Verification items for the finished model (mm, model axes). Face numbers are marked on the shaded views. A direction names the side the tool comes from. Coordinates: 2 decimals unless noted, no trailing zeros. Write each loop counter-clockwise with the first axis right and the second up, starting at its lowest first coordinate (ties: lowest second). Pieces come first, ordered by that corner, then holes. Notation, with made-up numbers: (25.5, 27) -> (80.5, 27) arc R24 cw to (80.5, 45) -> close; hole circle Ø9 at (8, 75.25). An arc over 180 degrees is marked (long way). Write item = value, one per line. Start each with the question number.
(1) Mould release check, pull along X, two halves, no side actions. Record for the marked faces 1, 2 and 3: released by +X, released by -X, zero draft, split by the parting line, or undercut.
(2) Gauge pin test, flat ends, axial feed: pin 1 Ø5 at (x, z) = (145, -8) entering from +Y; pin 2 Ø8 at (x, y) = (153.5, 53.5) entering from -Z; pin 3 Ø6 at (x, z) = (201.5, -1) entering from -Y; pin 4 Ø4 at (x, y) = (127.5, 61.5) entering from +Z. Record the tip position at first contact, or that the pin passes through.
(3) Material ranges on probe 1 along X at (y, z) = (67.25, 0); probe 2 along Z at (x, y) = (200, 43); probe 3 along X at (y, z) = (-4, 0), recorded low to high. Write a range as [from, to].
(4) Section check D-D (x = 59). Record the cut outline in (y, z) (3 decimals).
(5) Section check C-C (y = 57). Record the cut outline in (x, z), plus the area to 3 significant figures.
(6) Section check A-A (z = 0). Record the cut outline in (x, y), plus the area to 3 significant figures.
(7) Set-up check for the marked faces 4, 5, 6 and 7: record each of +Z, -Z, +X, -X, +Y, -Y from which the full face is reachable in a straight line by a thin tool's end or side.
(8) Section check B-B (x = 200). Record the cut outline in (y, z).
```python
from build123d import *

# Parameters (mm, degrees)
BOSS_EXTRUDE1_DEPTH     = 2
BOSS_EXTRUDE2_START     = -31.8
SKETCH3_W               = 60
SKETCH3_H               = 44
BOSS_EXTRUDE2_DEPTH     = 31.8
SKETCH4_R               = 4
BOSS_EXTRUDE3_DEPTH     = 7
CUT_EXTRUDE1_DEPTH      = 229.617169084
CUT_EXTRUDE1_DEPTH_BACK = 229.617169084
CUT_EXTRUDE2_DEPTH      = 228.560980838
CUT_EXTRUDE2_DEPTH_BACK = 228.560980838
SKETCH8_R               = 4.5
BOSS_EXTRUDE4_DEPTH     = 0.1


with BuildPart() as part:
    # Sketch1 → Boss-Extrude1 (new, symmetric)
    with BuildSketch(Plane.XY.offset(13.9)):
        Polygon((150, 27), (150, 71), (65.671641791, 44.328358209), (0, 0), (110, 0), align=None)
        Polygon((45.764296173, 14), (69.845614914, 30.25489015), (86.100505063, 14), align=None, mode=Mode.SUBTRACT)
        Polygon((84.347754219, 35.551740718), (136, 51.888477569), (136, 34.440899917), (105.826026877, 14.073468059), align=None, mode=Mode.SUBTRACT)
    extrude(amount=BOSS_EXTRUDE1_DEPTH, both=True)


with BuildPart() as body_2:
    # Mirror2: mirrored copy
    add(part.part.mirror(Plane.XY))


with BuildPart() as part_1:
    add(part.part)

    add(body_2.part)  # Boss-Extrude2 merges body 2
    # Sketch3 → Boss-Extrude2 (add)
    with BuildSketch(Plane.XY.offset(15.9).offset(BOSS_EXTRUDE2_START)):
        with Locations((180, 49)):
            Rectangle(SKETCH3_W, SKETCH3_H)
    extrude(amount=BOSS_EXTRUDE2_DEPTH)

    # Sketch4 → Boss-Extrude3 (add)
    with BuildSketch(Plane(origin=(0, 0, 0), x_dir=(1, 0, 0), z_dir=(0, 1, 0))):
        with BuildLine():
            Line((108.3763786, 39.867312377), (-1.6236214, 21.767312377))
            ThreePointArc((-1.6236214, 21.767312377), (-7.623523267, 18.37162213), (-10, 11.9))
            Line((-10, 11.9), (-10, -11.9))
            ThreePointArc((-10, -11.9), (-7.623523267, -18.37162213), (-1.6236214, -21.767312377))
            Line((-1.6236214, -21.767312377), (108.3763786, -39.867312377))
            ThreePointArc((108.3763786, -39.867312377), (116.47162213, -37.623523267), (120, -30))
            Line((120, -30), (120, 30))
            ThreePointArc((120, 30), (116.47162213, 37.623523267), (108.3763786, 39.867312377))
        make_face()
        with Locations(Location((110, 30, 0), (0, 0, 270))):
            Circle(SKETCH4_R, mode=Mode.SUBTRACT)
        with Locations(Location((110, -30, 0), (0, 0, 270))):
            Circle(SKETCH4_R, mode=Mode.SUBTRACT)
        with Locations(Location((0, 0, 0), (0, 0, 270))):
            Circle(SKETCH4_R, mode=Mode.SUBTRACT)
    extrude(amount=-BOSS_EXTRUDE3_DEPTH)

    # Sketch7 → Cut-Extrude1 (cut, two sides: drawn at the far end of the back side and taken through both)
    with BuildSketch(Plane.XY.offset(15.9).offset(-CUT_EXTRUDE1_DEPTH_BACK)):
        with BuildLine():
            Line((189.966629547, 50), (210, 50))
            Line((210, 50), (210, 48))
            Line((210, 48), (189.966629547, 48))
            ThreePointArc((189.966629547, 48), (160, 49), (189.966629547, 50))
        make_face()
    extrude(amount=CUT_EXTRUDE1_DEPTH + CUT_EXTRUDE1_DEPTH_BACK, mode=Mode.SUBTRACT)

    # Sketch8 → Cut-Extrude2 (cut, two sides: drawn at the far end of the back side and taken through both)
    with BuildSketch(Plane(origin=(0, 71, 0), x_dir=(1, 0, 0), z_dir=(0, 1, 0)).offset(-CUT_EXTRUDE2_DEPTH_BACK)):
        with Locations(Location((200, 0, 0), (0, 0, 270))):
            Circle(SKETCH8_R)
    extrude(amount=CUT_EXTRUDE2_DEPTH + CUT_EXTRUDE2_DEPTH_BACK, mode=Mode.SUBTRACT)

    # Sketch9 → Boss-Extrude4 (add)
    with BuildSketch(Plane.XY.offset(15.9)):
        with BuildLine():
            Line((150, 71), (150, 27))
            Line((150, 27), (210, 27))
            Line((210, 27), (210, 48))
            Line((210, 48), (189.966629547, 48))
            ThreePointArc((189.966629547, 48), (160, 49), (189.966629547, 50))
            Line((189.966629547, 50), (210, 50))
            Line((210, 50), (210, 71))
            Line((210, 71), (150, 71))
        make_face()
    extrude(amount=BOSS_EXTRUDE4_DEPTH)


solid = part_1.part
```
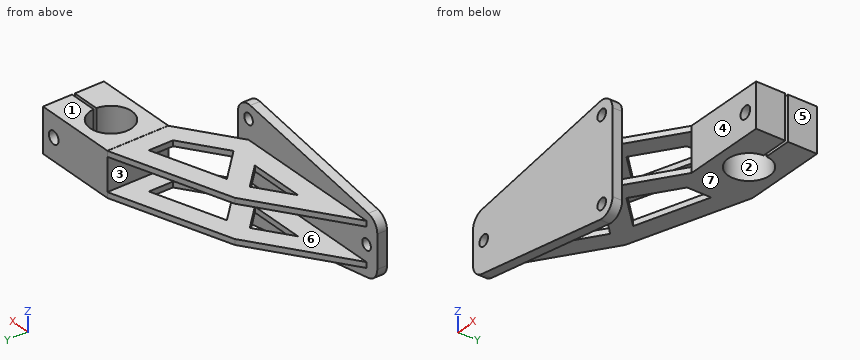
Response:
q1.face_1 = zero draft
q1.face_2 = undercut
q1.face_3 = released by -X
q2.pin_1 = through
q2.pin_2 = -15.9
q2.pin_3 = 27
q2.pin_4 = 15.9
q3.probe_1 = [150, 195.5], [204.5, 210]
q3.probe_2 = [-15.9, -4.5], [4.5, 16]
q3.probe_3 = [-10, -4], [4, 120]
q4.outline = (-7, -31.743) -> (0, -31.743) -> (0, -15.9) -> (14, -15.9) -> (14, -11.9) -> (0, -11.9) -> (0, 11.9) -> (14, 11.9) -> (14, 15.9) -> (0, 15.9) -> (0, 31.743) -> (-7, 31.743) -> close; (22.934, -15.9) -> (39.825, -15.9) -> (39.825, -11.9) -> (22.934, -11.9) -> close; (22.934, 11.9) -> (39.825, 11.9) -> (39.825, 15.9) -> (22.934, 15.9) -> close
q5.outline = (105.74, -15.9) -> (162.31, -15.9) -> (162.31, 16) -> (150, 16) -> (150, 15.9) -> (105.74, 15.9) -> (105.74, 11.9) -> (150, 11.9) -> (150, -11.9) -> (105.74, -11.9) -> close; (187.69, -15.9) -> (210, -15.9) -> (210, 16) -> (187.69, 16) -> close; hole circle Ø9 at (200, 0)
q5.area = 1,390 mm2
q6.outline = (-10, -7) -> (-4, -7) -> (-4, 0) -> (-10, 0) -> close; (4, -7) -> (120, -7) -> (120, 0) -> (4, 0) -> close; (150, 27) -> (195.5, 27) -> (195.5, 48) -> (189.97, 48) arc R15 cw (long way) to (189.97, 50) -> (195.5, 50) -> (195.5, 71) -> (150, 71) -> close; (204.5, 27) -> (210, 27) -> (210, 48) -> (204.5, 48) -> close; (204.5, 50) -> (210, 50) -> (210, 71) -> (204.5, 71) -> close
q6.area = 2,370 mm2
q7.face_4 = +Z, -Z, +X, -Y
q7.face_5 = +Z, -Z, +X, +Y, -Y
q7.face_6 = -X, +Y
q7.face_7 = -Z, +X, -X, +Y
q8.outline = (27, -15.9) -> (48, -15.9) -> (48, -4.5) -> (27, -4.5) -> close; (27, 4.5) -> (48, 4.5) -> (48, 16) -> (27, 16) -> close; (50, -15.9) -> (71, -15.9) -> (71, -4.5) -> (50, -4.5) -> close; (50, 4.5) -> (71, 4.5) -> (71, 16) -> (50, 16) -> close
